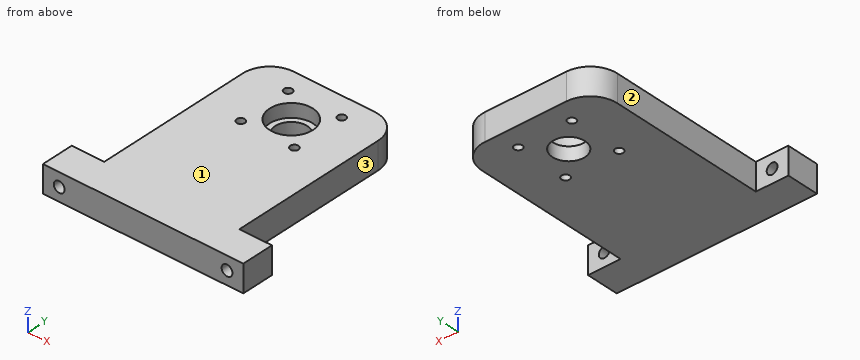
```python
from build123d import *

# Parameters (mm, degrees)
BOSS_EXTRUDE1_DEPTH = 10
SKETCH2_R           = 8
CUT_EXTRUDE1_DEPTH  = 5
FILLET1_R           = 10
SKETCH4_R           = 2
CUT_EXTRUDE3_DEPTH  = 21
SKETCH5_R           = 2
CUT_EXTRUDE4_DEPTH  = 25
SKETCH6_R           = 1.5
CUT_EXTRUDE5_DEPTH  = 10
CIRPATTERN1_COUNT   = 4
SKETCH8_R           = 6
CUT_EXTRUDE8_DEPTH  = 10


with BuildPart() as part:
    # Sketch1 → Boss-Extrude1 (new body)
    with BuildSketch(Plane.XY):
        Polygon((-37.625, -24), (36.375, -24), (36.375, -12), (24.375, -12), (24.375, 56), (-25.625, 56), (-25.625, -12), (-37.625, -12), align=None)
    extrude(amount=BOSS_EXTRUDE1_DEPTH)

    # Sketch2 → Cut-Extrude1 (cut)
    with BuildSketch(Plane.XY.offset(10)):
        with Locations((-0.625, 38)):
            Circle(SKETCH2_R)
    extrude(amount=-CUT_EXTRUDE1_DEPTH, mode=Mode.SUBTRACT)

    # Fillet1
    fillet1_edges = [part.edges().sort_by_distance(p)[0] for p in [
        (24.375, 56, 5),
        (-25.625, 56, 5),
    ]]
    fillet(fillet1_edges, radius=FILLET1_R)

    # Sketch4 → Cut-Extrude3 (cut)
    with BuildSketch(Plane(origin=(0, -12, 0), x_dir=(1, 0, 0), z_dir=(0, 1, 0))):
        with Locations(Location((30.375, -5, 0), (0, 0, 180))):
            Circle(SKETCH4_R)
    extrude(amount=-CUT_EXTRUDE3_DEPTH, mode=Mode.SUBTRACT)

    # Sketch5 → Cut-Extrude4 (cut)
    with BuildSketch(Plane(origin=(0, -12, 0), x_dir=(1, 0, 0), z_dir=(0, 1, 0))):
        with Locations(Location((-31.625, -5, 0), (0, 0, 270))):
            Circle(SKETCH5_R)
    extrude(amount=-CUT_EXTRUDE4_DEPTH, mode=Mode.SUBTRACT)

    # Sketch6 → Cut-Extrude5 (cut)
    with BuildSketch(Plane.XY.offset(10)):
        with Locations((9.274494937, 47.899494937)):
            Circle(SKETCH6_R)
    cut_extrude5 = extrude(amount=-CUT_EXTRUDE5_DEPTH, mode=Mode.SUBTRACT)

    # CirPattern1: Cut-Extrude5 ×4 about axis
    cirpattern1_axis = Axis((-0.625, 38, 0), (0, 0, 1))
    for i in range(1, CIRPATTERN1_COUNT):
        add(cut_extrude5.rotate(cirpattern1_axis, i * 360 / CIRPATTERN1_COUNT), mode=Mode.SUBTRACT)

    # Sketch8 → Cut-Extrude8 (cut)
    with BuildSketch(Plane.XY.offset(10)):
        with Locations((-0.625, 38)):
            Circle(SKETCH8_R)
    extrude(amount=-CUT_EXTRUDE8_DEPTH, mode=Mode.SUBTRACT)


solid = part.part
```
CAD build for the part. Positions are in the model's coordinates, mm. Face numbers are marked on the shaded views. A direction names the side the tool comes from. Round coordinates to 2 decimals unless told otherwise and drop trailing zeros. Write each loop counter-clockwise with the first axis right and the second up, starting at its lowest first coordinate (ties: lowest second). Pieces come first, ordered by that corner, then holes. Notation, with made-up numbers: (-14.5, 2.5) - (14.5, 2.5) arc R20 cw to (14.5, 18.5) - close; hole circle Ø2 at (-32.75, 17.5). An arc over 180 degrees is marked (long way). Return JSON: item names as keys, results as strings. Group by question number.
Item 1: Band-saw the part on B-B on x = 3. List the corners of the cut face in (y, z).
Item 2: Flat gauge pins, fed straight in: pin 1 Ø1.5 at (x, z) = (26, 2) entering from +Y; pin 2 Ø1 at (y, z) = (0.5, 3.5) entering from -X (3 decimals). Where does each tip first touch, or does it go through?
Item 3: Band-saw the part on C-C on z = 8.75. List the corners of the cut face in (x, y) (1 decimal).
Item 4: Probe probe 1 along Y at (x, z) = (33, 1.25); probe 2 along X at (y, z) = (-5, 9.25) (3 decimals); probe 3 along Y at (x, z) = (14.5, 1.25). List the from-to ranges inside material, lowest first.
Item 5: Band-saw the part on D-D on y = 15.5. List the corners of the cut face in (x, z) (3 decimals).
Item 6: Band-saw the part on A-A on y = 38. List the corners of the cut face in (x, z) (3 decimals), plus the area to 3 significant figures.
Item 7: 3-axis set-ups, long thin cutter, end or side, ignore diameter. For the marked faces 1, 2 and 3: which of +Z, -Z, +X, -X, +Y, -Y reach the whole face in a straight line?
Resolved:
{
 "1": {"outline": "(-24, 0) - (33.22, 0) - (33.22, 5) - (30.87, 5) - (30.87, 10) - (-24, 10) - close; (42.78, 0) - (56, 0) - (56, 10) - (45.13, 10) - (45.13, 5) - (42.78, 5) - close"},
 "2": {"pin 1": "stops at y = -12", "pin 2": "stops at x = -25.625"},
 "3": {"outline": "(-37.6, -24) - (36.4, -24) - (36.4, -12) - (24.4, -12) - (24.4, 46) arc R10 ccw to (14.4, 56) - (-15.6, 56) arc R10 ccw to (-25.6, 46) - (-25.6, -12) - (-37.6, -12) - close; hole circle Ø3 at (-10.5, 28.1); hole circle Ø3 at (-10.5, 47.9); hole circle Ø16 at (-0.6, 38); hole circle Ø3 at (9.3, 28.1); hole circle Ø3 at (9.3, 47.9)"},
 "4": {"probe 1": "y = -24 to -12", "probe 2": "x = -25.625 to 24.375", "probe 3": "y = -24 to 56"},
 "5": {"outline": "(-25.625, 0) - (24.375, 0) - (24.375, 10) - (-25.625, 10) - close"},
 "6": {"outline": "(-25.625, 0) - (-6.625, 0) - (-6.625, 5) - (-8.625, 5) - (-8.625, 10) - (-25.625, 10) - close; (5.375, 0) - (24.375, 0) - (24.375, 10) - (7.375, 10) - (7.375, 5) - (5.375, 5) - close", "area": "360 mm²"},
 "7": {"face 1": "+Z, +X, -X, +Y, -Y", "face 2": "+Z, -Z, -X, +Y", "face 3": "+Z, -Z, +X, +Y"}
}
